```python
from build123d import *

# Parameters (mm, degrees)
F0_W     = 131.804712
F0_H     = 138.758264
F1_DEPTH = 173.228
F3_DEPTH = 11.684


with BuildPart() as f1:
    # F0 (on Right) → F1 (new body)
    with BuildSketch(Plane.YZ):
        with Locations((42.563114, -6.31338)):
            Rectangle(F0_W, F0_H)
    extrude(amount=F1_DEPTH)

    # F2 (on face) → F3 (join)
    with BuildSketch(Plane(origin=(0, 0, -75.692512), x_dir=(1, 0, 0), z_dir=(0, 0, -1))):
        Polygon((108.57549, -52.235217), (117.505729, -42.851768), (88.673443, -12.412787), (72.527371, -10.27096), (74.174926, -23.451431), align=None)
        Polygon((130.027175, -68.100274), (137.895701, -59.610553), (120.636091, -47.835302), (124.036072, -42.851768), (117.505729, -42.851768), (108.57549, -52.235217), (106.961355, -53.93127), (108.57549, -59.457818), (112.233534, -54.096028), align=None)
    extrude(amount=F3_DEPTH)


solid = f1.part
```
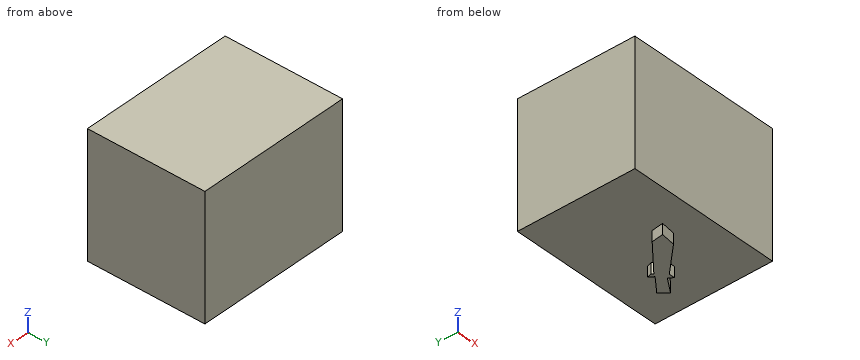
For this review, take the finished solid that the model builds, in its own axes (mm). Round coordinates to 2 decimals unless told otherwise and drop trailing zeros. Write each loop counter-clockwise with the first axis right and the second up, starting at its lowest first coordinate (ties: lowest second). Pieces come first, ordered by that corner, then holes. Notation, with made-up numbers: (-34, -4.75) -> (6, -4.75) arc R21 ccw to (6, 18.25) -> close; hole circle Ø9 at (27, 29). An arc over 180 degrees is marked (long way). One line per question, with ' | ' between items. Start each with the question number.
(1) Add section A-A, the plane y = 94. Write out the cut boundary in (x, z).
(2) Insertion check: P1, Ø2, axis at x = 122, z = -81, coming from the -Y side; P2, Ø6, axis at x = 25.5, y = 92, coming from the -Z side. Each pin has a flat end and moves straight along its axis. Give the tip position at first contact, or say it passes through.
(3) Add section B-B, the plane x = 24. Write out the cut boundary in (y, z), plus the area to 3 significant figures.
(4) For line 1 along Z through (x, y) = (126, 80), list the stretches that pass through material, from the lowest coordinate up. Write a range as from..to.
Answer list:
1) outline: (0, -75.69) -> (173.23, -75.69) -> (173.23, 63.07) -> (0, 63.07) -> close
2) P1: y = 42.85 | P2: z = -75.69
3) outline: (-23.34, -75.69) -> (108.47, -75.69) -> (108.47, 63.07) -> (-23.34, 63.07) -> close | area: 18,300 mm²
4) line 1: -75.69..63.07
